The figure shows three views and two pictorial views of one solid part (mm, origin at its lowest corner). Answer the questions. A direction names the side the tool comes from. Coordinates: 2 decimals unless noted, no trailing zeros. Order: outer loops, then holes, each group sorted by start corner. A loop starts at its lowest first (then second) coordinate and runs counter-clockwise, first axis right, second up. Notation, with made-up numbers: (60, 47) -> (89, 47) arc R28 cw to (89, 74) -> close; hole circle Ø8 at (30.5, 41). An arc over 180 degrees is marked (long way). Return JSON: item names as keys, results as strings. Group by question number.
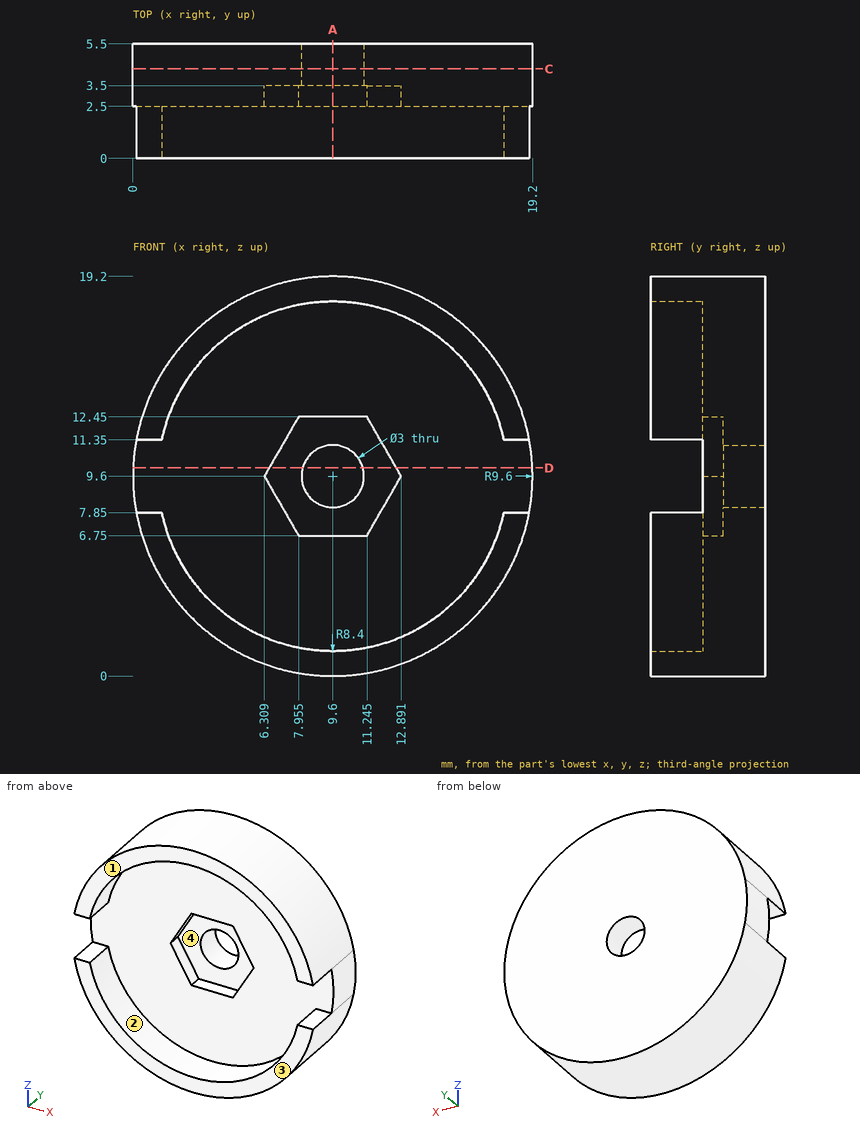
1. Which of the six approach directions +Z, -Z, +X, -X, +Y, -Y give full straight-line access (tool end or side, diameter ignored) to the marked faces 1 and 2?
2. Find section C-C on y = 4.3. Determine the outline of the cut face in (x, z).
3. Straight lines are drawn through the part: L1, parallel to Z at x = 9.6, y = 4.85; L2, parallel to Y at x = 3, z = 5.25; L3, parallel to X at y = 1.85, z = 5 (1 decimal). For each, find the intervals that lie inside material, in ascending order.
4. Find section D-D on z = 10. Determine the outline of the cut face in (x, y) (1 decimal).
5. For a pull along X with two mould halves and no side action, classify the marked faces 3 and 4 as released by +X, released by -X, zero draft, split by the parting line, or undercut.
6. Given pin 1 (8 mm diameter, centred on x = 8, z = 3.5, fed in from -Y); pin 2 (1.5 mm diameter, centred on y = 1, z = 15, fed in from -X); pin 3 (1.3 mm diameter, centred on x = 1, y = 1, fed in from -Z); pin 4 (0.6 mm diameter, centred on x = 18.5, y = 1, fed in from +Z) (1 decimal), each flat-ended and moving along its own axis, determine where each tip first touches the part or whether it passes through.
7. Find section A-A on x = 9.6. Determine the outline of the cut face in (y, z).
Result:
{
 "1": {"face 1": "+Z, -Z, +X, -X, -Y", "face 2": "-Y"},
 "2": {"outline": "circle Ø19.2 at (9.6, 9.6); hole circle Ø3 at (9.6, 9.6)"},
 "3": {"L1": "0 to 8.1, 11.1 to 19.2", "L2": "2.5 to 5.5", "L3": "1.2 to 2.6, 16.6 to 18"},
 "4": {"outline": "(0, 2.5) -> (6.5, 2.5) -> (6.5, 3.5) -> (8.2, 3.5) -> (8.2, 5.5) -> (0, 5.5) -> close; (11, 3.5) -> (12.7, 3.5) -> (12.7, 2.5) -> (19.2, 2.5) -> (19.2, 5.5) -> (11, 5.5) -> close"},
 "5": {"face 3": "zero draft", "face 4": "undercut"},
 "6": {"pin 1": "y = 0", "pin 2": "x = 1.2", "pin 3": "z = 4.22", "pin 4": "z = 13.9"},
 "7": {"outline": "(0, 0) -> (5.5, 0) -> (5.5, 8.1) -> (3.5, 8.1) -> (3.5, 6.75) -> (2.5, 6.75) -> (2.5, 1.2) -> (0, 1.2) -> close; (0, 18) -> (2.5, 18) -> (2.5, 12.45) -> (3.5, 12.45) -> (3.5, 11.1) -> (5.5, 11.1) -> (5.5, 19.2) -> (0, 19.2) -> close"}
}
